Source: three-view drawing plus pictorial views. Frame: mm from the lowest corner of the part. Give positions to 0.01 mm unless a question says otherwise; leave off trailing zeros. Order: outer loops, then holes, each group sorted by start corner. A loop starts at its lowest first (then second) coordinate and runs counter-clockwise, first axis right, second up. Notation, with made-up numbers: (30, -18.75) -> (38, -18.75) arc R35 cw to (38, 19.25) -> close; hole circle Ø9 at (33.5, 12). An arc over 180 degrees is marked (long way). Answer in a Markdown table with one row per item.
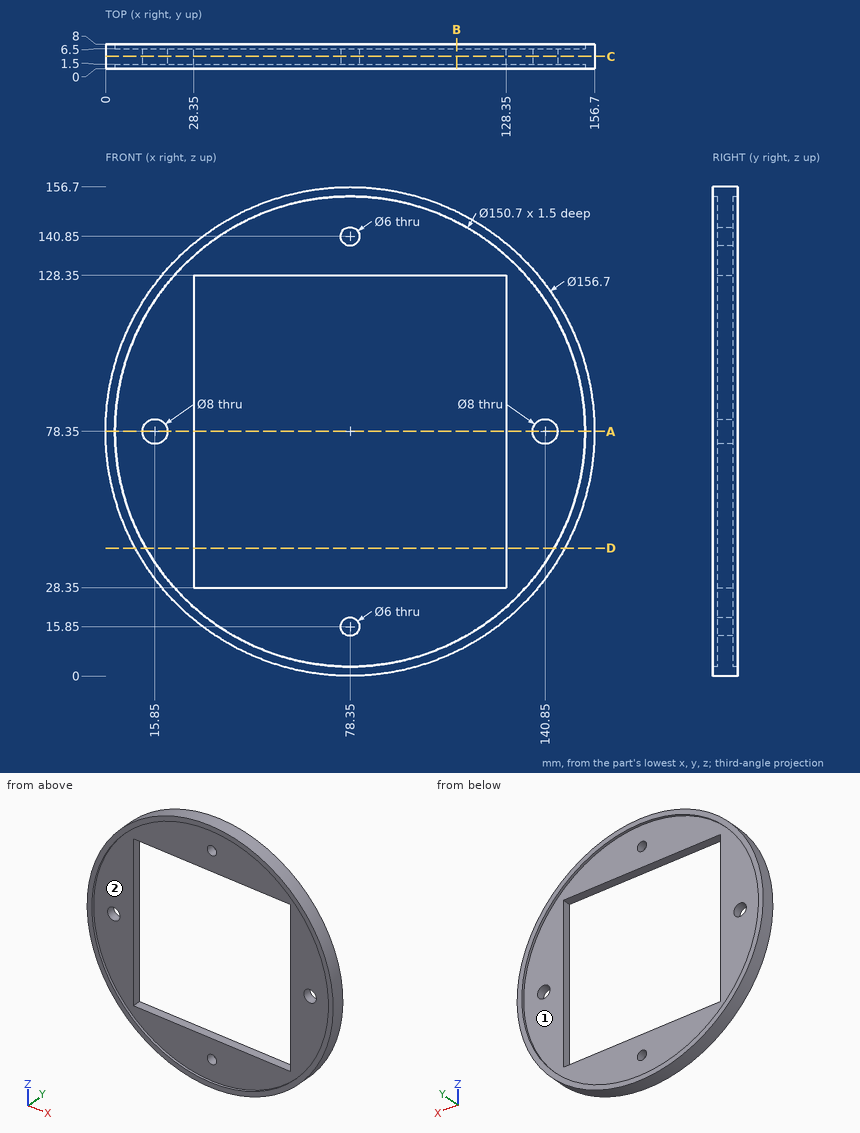
(1) Pull-direction query (Z, two-part tool) for the marked faces 1 and 2; classes: +Z half, -Z half, draft (parallel to the pull), parting line (faces both ways), or undercut.
A:
| item | result |
|---|---|
| face 1 | undercut |
| face 2 | undercut |
(2) Ray query, probe 1 along X at (y, z) = (4.7, 78.35); probe 2 along X at (y, z) = (0.9, 78.35); probe 3 along Y at (x, z) = (134.5, 42.5). Return the intervals inside material, ascending.
A:
| item | result |
|---|---|
| probe 1 | x = 0 to 11.85, 19.85 to 28.35, 128.35 to 136.85, 144.85 to 156.7 |
| probe 2 | x = 0 to 3, 153.7 to 156.7 |
| probe 3 | y = 1.5 to 6.5 |
(3) Section query C-C (y = 4). Return the cut outline in (x, z).
A:
| item | result |
|---|---|
| outline | circle Ø156.7 at (78.35, 78.35); hole circle Ø8 at (15.85, 78.35); hole (28.35, 28.35) -> (128.35, 28.35) -> (128.35, 128.35) -> (28.35, 128.35) -> close; hole circle Ø6 at (78.35, 15.85); hole circle Ø6 at (78.35, 140.85); hole circle Ø8 at (140.85, 78.35) |
(4) Section query B-B (x = 112.5). Return the cut outline in (y, z), plus the area to 3 significant figures.
A:
| item | result |
|---|---|
| outline | (0, 7.83) -> (8, 7.83) -> (8, 11.18) -> (6.5, 11.18) -> (6.5, 28.35) -> (1.5, 28.35) -> (1.5, 11.18) -> (0, 11.18) -> close; (0, 145.52) -> (1.5, 145.52) -> (1.5, 128.35) -> (6.5, 128.35) -> (6.5, 145.52) -> (8, 145.52) -> (8, 148.87) -> (0, 148.87) -> close |
| area | 225 mm^2 |
(5) First-contact query: pin 1 Ø6 at (x, z) = (31, 87.5) entering from +Y; pin 2 Ø4 at (y, z) = (4, 82) entering from +X; pin 3 Ø7 at (x, z) = (78.35, 15.85) entering from -Y. Flat tips, straight axial feed; report the tip coordinate or a pass-through.
A:
| item | result |
|---|---|
| pin 1 | stops at y = 6.5 |
| pin 2 | stops at x = 156.68 |
| pin 3 | stops at y = 1.5 |
(6) Section query A-A (z = 78.35). Return the cut outline in (x, y).
A:
| item | result |
|---|---|
| outline | (0, 0) -> (3, 0) -> (3, 1.5) -> (11.85, 1.5) -> (11.85, 6.5) -> (3, 6.5) -> (3, 8) -> (0, 8) -> close; (19.85, 1.5) -> (28.35, 1.5) -> (28.35, 6.5) -> (19.85, 6.5) -> close; (128.35, 1.5) -> (136.85, 1.5) -> (136.85, 6.5) -> (128.35, 6.5) -> close; (144.85, 1.5) -> (153.7, 1.5) -> (153.7, 0) -> (156.7, 0) -> (156.7, 8) -> (153.7, 8) -> (153.7, 6.5) -> (144.85, 6.5) -> close |
(7) Section query D-D (z = 41). Return the cut outline in (x, y).
A:
| item | result |
|---|---|
| outline | (9.48, 0) -> (12.91, 0) -> (12.91, 1.5) -> (28.35, 1.5) -> (28.35, 6.5) -> (12.91, 6.5) -> (12.91, 8) -> (9.48, 8) -> close; (128.35, 1.5) -> (143.79, 1.5) -> (143.79, 0) -> (147.22, 0) -> (147.22, 8) -> (143.79, 8) -> (143.79, 6.5) -> (128.35, 6.5) -> close |
